from build123d import *

# Parameters (mm, degrees)
SKETCH1_W                = 20
SKETCH1_H                = 6
BOSS_EXTRUDE1_DEPTH      = 2.5
SKETCH2_R                = 0.95
BOSS_EXTRUDE2_DEPTH      = 2.5
BOSS_EXTRUDE2_DEPTH_BACK = 8.5
SKETCH4_W                = 5.869913051
SKETCH4_H                = 6
BOSS_EXTRUDE3_DEPTH      = 7


with BuildPart() as part:
    # Sketch1 → Boss-Extrude1 (new body)
    with BuildSketch(Plane(origin=(0, 0, 0), x_dir=(1, 0, 0), z_dir=(0, 1, 0))):
        Rectangle(SKETCH1_W, SKETCH1_H)
    extrude(amount=BOSS_EXTRUDE1_DEPTH)

    # Sketch2 → Boss-Extrude2 (add, two sides)
    with BuildSketch(Plane.XY.offset(3)) as boss_extrude2_sk:
        with Locations((8, 1.25)):
            Circle(SKETCH2_R)
    extrude(amount=BOSS_EXTRUDE2_DEPTH)
    extrude(boss_extrude2_sk.sketch, amount=-BOSS_EXTRUDE2_DEPTH_BACK)

    # Sketch4 → Boss-Extrude3 (add)
    with BuildSketch(Plane(origin=(0, 2.5, 0), x_dir=(1, 0, 0), z_dir=(0, 1, 0))):
        with Locations((-7.065043474, 0)):
            Rectangle(SKETCH4_W, SKETCH4_H)
    extrude(amount=BOSS_EXTRUDE3_DEPTH)


solid = part.part
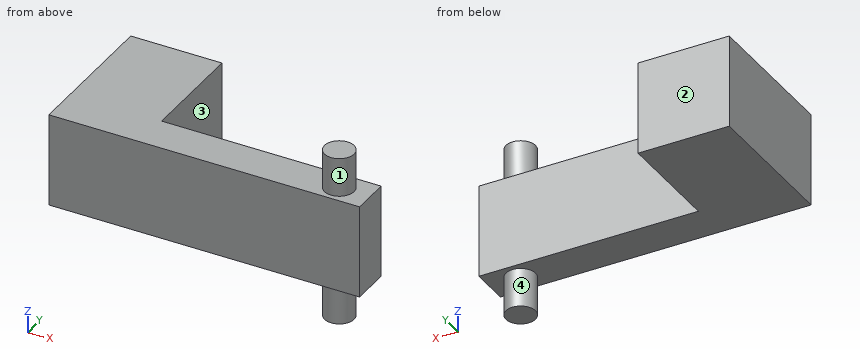
CAD build for the part. Positions are in the model's coordinates, mm. Face numbers are marked on the shaded views. A direction names the side the tool comes from. Give positions to 0.01 mm unless a question says otherwise; leave off trailing zeros. Write each loop counter-clockwise with the first axis right and the second up, starting at its lowest first coordinate (ties: lowest second). Pieces come first, ordered by that corner, then holes. Notation, with made-up numbers: (76.5, 28.5) - (107.5, 28.5) arc R18 cw to (107.5, 34.5) - close; hole circle Ø4 at (85, -12.5). An arc over 180 degrees is marked (long way). Put each result on its own line as item: value.
(1) Wall check: L1, parallel to X at y = 7, z = -0.75; L2, parallel to Z at x = -6.5, y = 1; L3, parallel to Y at x = 0.25, z = 2.5. Give the ranges that are in metal, low to high.
Working result:
L1: -10 to -4.13
L2: -3 to 3
L3: 0 to 2.5
(2) Saw through at A-A (z = 2). List the corners of the cut face in (x, y).
Working result:
outline: (-10, 0) - (10, 0) - (10, 2.5) - (-4.13, 2.5) - (-4.13, 9.5) - (-10, 9.5) - close
(3) Tool access for the marked faces 1, 2, 3 and 4: list every direction of +Z, -Z, +X, -X, +Y, -Y with a clear straight run to the whole face (end or side of a thin tool).
Working result:
face 1: +Z
face 2: +Z, -Z, +X, -X, +Y
face 3: +Z, -Z, +X, +Y
face 4: -Z
(4) Saw through at D-D (y = 4.75). List the corners of the cut face in (x, z), then the cut area to 3 significant figures.
Working result:
outline: (-10, -3) - (-4.13, -3) - (-4.13, 3) - (-10, 3) - close
area: 35.2 mm^2
(5) Saw through at B-B (x = 8). List the corners of the cut face in (y, z), then the cut area to 3 significant figures.
Working result:
outline: (0, -3) - (0.3, -3) - (0.3, -5.5) - (2.2, -5.5) - (2.2, -3) - (2.5, -3) - (2.5, 3) - (2.2, 3) - (2.2, 5.5) - (0.3, 5.5) - (0.3, 3) - (0, 3) - close
area: 24.5 mm^2
(6) Saw through at C-C (y = 1.25). List the corners of the cut face in (x, z).
Working result:
outline: (-10, -3) - (7.05, -3) - (7.05, -5.5) - (8.95, -5.5) - (8.95, -3) - (10, -3) - (10, 3) - (8.95, 3) - (8.95, 5.5) - (7.05, 5.5) - (7.05, 3) - (-10, 3) - close
(7) Drop flat-ended pins along their axis: pin 1 Ø3 at (x, z) = (3.5, -1) entering from +Y; pin 2 Ø5 at (x, y) = (-5, 4.5) entering from +Z; pin 3 Ø1.8 at (y, z) = (7.5, 0) entering from +X; pin 4 Ø5 at (y, z) = (5.5, 3.5) entering from -X. Give the stop position or say it passes through.
Working result:
pin 1: y = 2.5
pin 2: z = 3
pin 3: x = -4.13
pin 4: x = -10
